from build123d import *

# Parameters (mm, degrees)
SKETCH1_R             = 11
SKETCH1_R_2           = 9.5
BOSS_EXTRUDE1_DEPTH   = 7
SKETCH1_R_3           = 6
SKETCH1_R_4           = 4
BOSS_EXTRUDE1_2_DEPTH = 7
BOSS_EXTRUDE2_START   = -6.4
SKETCH2_R             = 9.5
SKETCH2_R_2           = 6
BOSS_EXTRUDE2_DEPTH   = 6.4
CHAMFER1_SIZE         = 0.2
CHAMFER2_SIZE         = 0.5


with BuildPart() as part:
    # Sketch1 → Boss-Extrude1 (new body)
    with BuildSketch(Plane(origin=(0, 0, 0), x_dir=(1, 0, 0), z_dir=(0, 1, 0))):
        with Locations(Location((0, 0, 0), (0, 0, 270))):
            Circle(SKETCH1_R)
        with Locations(Location((0, 0, 0), (0, 0, 270))):
            Circle(SKETCH1_R_2, mode=Mode.SUBTRACT)
    extrude(amount=BOSS_EXTRUDE1_DEPTH)



with BuildPart() as body_2:
    # Sketch1 → Boss-Extrude1 2 (new body)
    with BuildSketch(Plane(origin=(0, 0, 0), x_dir=(1, 0, 0), z_dir=(0, 1, 0))):
        with Locations(Location((0, 0, 0), (0, 0, 270))):
            Circle(SKETCH1_R_3)
        with Locations(Location((0, 0, 0), (0, 0, 270))):
            Circle(SKETCH1_R_4, mode=Mode.SUBTRACT)
    extrude(amount=BOSS_EXTRUDE1_2_DEPTH)


with BuildPart() as part_1:
    add(part.part)

    add(body_2.part)  # Boss-Extrude2 merges body 2
    # Sketch2 → Boss-Extrude2 (add)
    with BuildSketch(Plane(origin=(0, 6.7, 0), x_dir=(1, 0, 0), z_dir=(0, 1, 0)).offset(BOSS_EXTRUDE2_START)):
        with Locations(Location((0, 0, 0), (0, 0, 270))):
            Circle(SKETCH2_R)
        with Locations(Location((0, 0, 0), (0, 0, 270))):
            Circle(SKETCH2_R_2, mode=Mode.SUBTRACT)
    extrude(amount=BOSS_EXTRUDE2_DEPTH)

    # Chamfer1
    chamfer1_edges = [part_1.edges().sort_by_distance(p)[0] for p in [
        (0, 0, -6),
        (0, 7, -6),
        (0, 0, -9.5),
        (0, 7, -9.5),
    ]]
    chamfer(chamfer1_edges, length=CHAMFER1_SIZE)

    # Chamfer2
    chamfer2_edges = [part_1.edges().sort_by_distance(p)[0] for p in [
        (0, 7, -11),
        (0, 7, -4),
        (0, 0, -4),
        (0, 0, -11),
    ]]
    chamfer(chamfer2_edges, length=CHAMFER2_SIZE)


solid = part_1.part
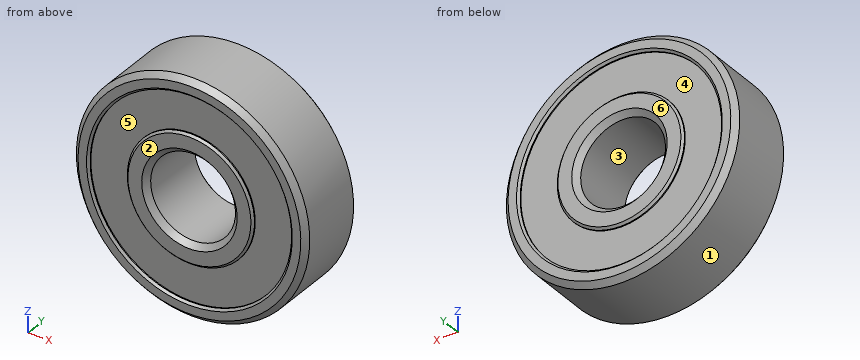
Model file for the job. Use its own axes, mm. Face numbers are marked on the shaded views. A direction names the side the tool comes from. Round coordinates to 2 decimals unless told otherwise and drop trailing zeros. Loops run counter-clockwise (first coordinate to the right, second up) from the corner with the lowest first, then second, coordinate; pieces in that order, holes last. Notation, with made-up numbers: (23.5, 55) -> (67.5, 55) arc R12 ccw to (67.5, 64) -> close; hole circle Ø6 at (79.5, 68.25). An arc over 180 degrees is marked (long way). Answer as CSV lines item,"result". Start each with the question number.
1) Slice it at A-A (y = 2.75). List the corners of the cut face in (x, z), plus the area to 3 significant figures.
2) Mould opens along Z. For the marked faces 1, 2, 3 and 4 say: +Z half, -Z half, draft (parallel to the pull), parting line (faces both ways), or undercut.
3) Pin check, flat tips, straight feed: P1, Ø4, axis at x = -7.5, y = 6, coming from the +Z side; P2, Ø6.5, axis at x = 0, z = 0, coming from the +Y side; P3, Ø1.5, axis at x = 7.5, y = 1.5, coming from the +Z side; P4, Ø1.5, axis at x = -4.5, y = 1, coming from the -Z side. Stop position of each tip, or through.
4) Probe line 1 along Z through (x, y) = (-3.25, 6.75); line 2 along X through (y, z) = (1.7, 0); line 3 along X through (y, z) = (3.5, 3). List the from-to ranges inside material, lowest first.
5) Tool access for the marked faces 5 and 6: list every direction of +Z, -Z, +X, -X, +Y, -Y with a clear straight run to the whole face (end or side of a thin tool).
Filled in:
1,outline,"circle Ø22 at (0, 0); hole circle Ø8 at (0, 0)"
1,area,"330 mm2"
2,face 1,"parting line"
2,face 2,"draft"
2,face 3,"undercut"
2,face 4,"undercut"
3,P1,"stops at z = 9.53"
3,P2,"passes through"
3,P3,"stops at z = 8.69"
3,P4,"stops at z = -10.34"
4,line 1,"z = -10.25 to -8.93, -5.04 to -2.74, 2.74 to 5.04, 8.93 to 10.25"
4,line 2,"x = -11 to -4, 4 to 11"
4,line 3,"x = -10.58 to -2.65, 2.65 to 10.58"
5,face 5,"-Y"
5,face 6,"+Z, -Z, +X, -X, +Y"
